Can you work these out from the model? Positions are in its coordinate system, mm. A direction names the side the tool comes from. Coordinates: 2 decimals unless noted, no trailing zeros. Order: outer loops, then holes, each group sorted by start corner. A loop starts at its lowest first (then second) coordinate and runs counter-clockwise, first axis right, second up. Notation, with made-up numbers: (20.5, 1.25) - (31.5, 1.25) arc R25 cw to (31.5, 26.25) - close; hole circle Ø8 at (-10.5, -25). An arc over 180 degrees is marked (long way). Return JSON: item names as keys, results as strings. Group by question number.
1) Imagine slicing it at B-B (x = 3.25). Write out the boundary of the cut face in (y, z).
2) Imagine slicing it at A-A (y = 4). Write out the boundary of the cut face in (x, z), and give its area (3 significant figures).
3) For pin 1 Ø5 at (x, y) = (-5, 38) entering from +Z; pin 2 Ø5 at (x, y) = (-2, 28) entering from +Z, each with a flat end and sliding along its axis, tell me the tip position at first contact or that it passes through.
4) If I drill on line 1 along X through (y, z) = (16, 9); line 2 along Z through (x, y) = (-4, 20); line 3 along Z through (x, y) = (2.5, 18.5), over which ranges is the centre line in solid material (lowest first)?
5) If we mould it in two halves opening along X, with no side actions, what happens to faces 1 (the face through (-3.062, 28.052, 21.314)), 2 (the face through (0, 29, 15.93)), 3 (the face through (0, 0, 0))? For each: pulls with the +X half, pulls with the -X half, needs draft (parallel to the pull), parting line crosses it, or undercut.
6) Imagine slicing it at D-D (z = 18). Write out the boundary of the cut face in (x, y).
7) Which directions (+Z, -Z, +X, -X, +Y, -Y) give clear straight access to the entire face, cutting with the end or side of a thin tool? Please do faces 4 (the face through (-5, 29, 11)), 5 (the face through (-7, 28, 0)).
8) Imagine slicing it at C-C (z = 12.5). Write out the boundary of the cut face in (x, y), and give its area (3 significant figures).
```python
from build123d import *

# Parameters (mm, degrees)
SKETCH_2_W          = 14
SKETCH_2_H          = 52.3
EXTRUDE_1_DEPTH     = 56.9
SKETCH_3_W          = 5
SKETCH_3_H          = 5
CUT_EXTRUDE_1_DEPTH = 56.9
FILLET_6_R          = 15


with BuildPart() as part:
    # Эскиз2 → Бобышка-Вытянуть1 (new body)
    with BuildSketch(Plane(origin=(0, 0, 0), x_dir=(1, 0, 0), z_dir=(0, 1, 0))):
        Rectangle(SKETCH_2_W, SKETCH_2_H)
    extrude(amount=EXTRUDE_1_DEPTH)

    # Эскиз3 → Вырез-Вытянуть1 (cut)
    with BuildSketch(Plane(origin=(0, 56.9, 0), x_dir=(1, 0, 0), z_dir=(0, 1, 0))):
        with Locations((-2.5, -13.43)):
            Rectangle(SKETCH_3_W, SKETCH_3_H)
        with Locations((-2.5, -8.43)):
            Rectangle(SKETCH_3_W, SKETCH_3_H)
        with Locations((2.5, -8.43)):
            Rectangle(SKETCH_3_W, SKETCH_3_H)
        with Locations((2.5, -13.43)):
            Rectangle(SKETCH_3_W, SKETCH_3_H)
    extrude(amount=-CUT_EXTRUDE_1_DEPTH, mode=Mode.SUBTRACT)

    # Скругление6
    # the kernel refuses this fillet: 15 mm, written as the material it takes off along each edge
    with BuildSketch(Plane(origin=(-7, -37.416573868, -26.15), x_dir=(1, 0, 0), z_dir=(0, 1, 0))) as fillet_6_piece_1:
        with BuildLine():
            CenterArc((15, -14.966629547), FILLET_6_R, 93.822553729, 86.177446271)
            Line((0, -14.966629547), (-0.3, -14.966629547))
            Line((-0.3, -14.966629547), (-0.3, 0))
            Line((-0.3, 0), (0, 0.3))
            ThreePointArc((0, 0.3), (7, 0.3), (13.98, 0.299332591))
            Line((13.98, 0.299332591), (14, 0))
        make_face()
    extrude(amount=131.733147735, mode=Mode.SUBTRACT)
    with BuildSketch(Plane(origin=(-7, -37.416573868, 26.15), x_dir=(0, 0, -1), z_dir=(0, 1, 0))) as fillet_6_piece_2:
        with BuildLine():
            CenterArc((14.966629547, -15), FILLET_6_R, 90, 86.177446271)
            Line((0, -14), (-0.299332591, -13.98))
            ThreePointArc((-0.299332591, -13.98), (-0.3, -7), (-0.3, 0))
            Line((-0.3, 0), (0, 0.3))
            Line((0, 0.3), (14.966629547, 0.3))
            Line((14.966629547, 0.3), (14.966629547, 0))
        make_face()
    extrude(amount=131.733147735, mode=Mode.SUBTRACT)


solid = part.part
```
Calculated:
{
 "1": {"outline": "(0, -25.41) - (56.9, -25.41) - (56.9, 5.93) - (0, 5.93) - close; (0, 15.93) - (56.9, 15.93) - (56.9, 25.41) - (0, 25.41) - close"},
 "2": {"outline": "(-7, -11.18) arc R15 ccw to (7, -26.15) - (7, 26.15) arc R15 ccw to (-7, 11.18) - close; hole (-5, 5.93) - (5, 5.93) - (5, 15.93) - (-5, 15.93) - close", "area": "537 mm2"},
 "3": {"pin 1": "z = 21.9", "pin 2": "z = 24.17"},
 "4": {"line 1": "-7 to -5, 5 to 7", "line 2": "-20.18 to 5.93, 15.93 to 20.18", "line 3": "-25.14 to 5.93, 15.93 to 25.14"},
 "5": {"face 1": "pulls with the -X half", "face 2": "undercut", "face 3": "needs draft"},
 "6": {"outline": "(-5.36, 0) - (7, 0) - (7, 56.9) - (-5.36, 56.9) - close"},
 "7": {"face 4": "+Y, -Y", "face 5": "+Z, -Z, -X, +Y, -Y"},
 "8": {"outline": "(-6.94, 0) - (-5, 0) - (-5, 56.9) - (-6.94, 56.9) - close; (5, 0) - (7, 0) - (7, 56.9) - (5, 56.9) - close", "area": "224 mm2"}
}
